Geometry: final body of the model. Coordinates: model frame, mm. Round coordinates to 2 decimals unless told otherwise and drop trailing zeros. Write each loop counter-clockwise with the first axis right and the second up, starting at its lowest first coordinate (ties: lowest second). Pieces come first, ordered by that corner, then holes. Notation, with made-up numbers: M 40.25,40.25 L 54.25,40.25 A29 ccw 54.25,70.25 Z; hole C 24.5,78.25 d9. An arc over 180 degrees is marked long. Use one line per item in the form item = value. Start each with the question number.
Item 1: Ray query, probe 1 along Y at (x, z) = (0, -18); probe 2 along Y at (x, z) = (0.25, 17); probe 3 along X at (y, z) = (0, -38.5). Return the intervals inside material, ascending.
Item 2: Section query A-A (z = 47). Return loops of the section in (x, y), and give its area (3 significant figures).
Item 3: Pin query (flat end, axial travel): pin 1 Ø4.5 at (x, y) = (0, 0) entering from -Z; pin 2 Ø1.6 at (x, y) = (-5.5, 4) entering from -Z (3 decimals); pin 3 Ø1.5 at (x, z) = (-3, 21.5) entering from -Y. Return the tip coordinate at first contact, or that it passes through.
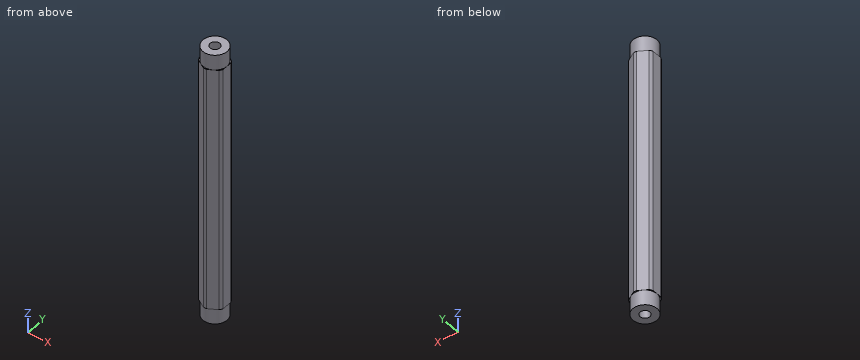
Autodesk Inventor part; units mm, degrees
ref_plane "YZ Plane" through (0, 0, 0) normal (1, 0, 0) x (0, 1, 0)
ref_plane "XZ Plane" through (0, 0, 0) normal (0, 1, 0) x (-1, 0, 0)
ref_plane "XY Plane" through (0, 0, 0) normal (0, 0, 1) x (1, 0, 0)
sketch "Sketch1" plane through (0, 0, 0) normal (0, 0, 1) x (1, 0, 0)
  line L0 (-6.35, -3.6662) -> (-6.35, 3.6662)
  line L1 (-6.35, 3.6662) -> (0, 7.3323)
  line L2 (0, 7.3323) -> (6.35, 3.6662)
  line L3 (6.35, 3.6662) -> (6.35, -3.6662)
  line L4 (6.35, -3.6662) -> (0, -7.3323)
  line L5 (0, -7.3323) -> (-6.35, -3.6662)
  point P0 (0, 0)
  point P1 (0, 0)
  dimension "Size" = 12.7
extrude "Extrusion1" add sketch "Sketch1" along normal mid plane 146.05
sketch "Sketch3" plane through (0, 0, 73.025) normal (0, 0, 1) x (1, 0, 0)
  line L0 (-6.35, 3.6662) -> (0, 7.3323) construction
  line L1 (0, 7.3323) -> (6.35, 3.6662) construction
  line L2 (6.35, 3.6662) -> (6.35, -3.6662) construction
  line L3 (6.35, -3.6662) -> (0, -7.3323) construction
  line L4 (0, -7.3323) -> (-6.35, -3.6662) construction
  line L5 (-6.35, -3.6662) -> (-6.35, 3.6662) construction
  point P0 (0, 0)
hole "Hole1" at (0, 0, 73.025) direction (0, 0, -1) diameter 5.1054 end through all
sketch "Sketch4" plane through (0, 0, 73.025) normal (0, 0, 1) x (1, 0, 0)
  circle A0 centre (0, 0) radius 2.5527 construction
  line L0 (-6.35, 3.6662) -> (0, 7.3323) construction
  line L1 (0, 7.3323) -> (6.35, 3.6662) construction
  line L2 (6.35, 3.6662) -> (6.35, -3.6662) construction
  line L3 (6.35, -3.6662) -> (0, -7.3323) construction
  line L4 (0, -7.3323) -> (-6.35, -3.6662) construction
  line L5 (-6.35, -3.6662) -> (-6.35, 3.6662) construction
  circle A1 centre (0, 0) radius 6.8771
  circle A2 centre (0, 0) radius 8.89
  dimension "thunder" = 13.7541
  dimension "d16" = 17.78
extrude "Extrusion3" cut sketch "Sketch4" against normal through all
sketch "Sketch5" plane through (0, 0, 73.025) normal (0, 0, 1) x (1, 0, 0)
  arc A0 (5.4616, -4.1791) -> (6.35, -2.6403) centre (0, 0) ccw
  line L0 (5.4616, -4.1791) -> (0.8884, -6.8194)
  arc A1 (-0.8884, -6.8194) -> (0.8884, -6.8194) centre (0, 0) ccw
  line L1 (-0.8884, -6.8194) -> (-5.4616, -4.1791)
  arc A2 (-6.35, -2.6403) -> (-5.4616, -4.1791) centre (0, 0) ccw
  line L2 (-6.35, -2.6403) -> (-6.35, 2.6403)
  arc A3 (-5.4616, 4.1791) -> (-6.35, 2.6403) centre (0, 0) ccw
  line L3 (-5.4616, 4.1791) -> (-0.8884, 6.8194)
  arc A4 (0.8884, 6.8194) -> (-0.8884, 6.8194) centre (0, 0) ccw
  line L4 (0.8884, 6.8194) -> (5.4616, 4.1791)
  arc A5 (6.35, 2.6403) -> (5.4616, 4.1791) centre (0, 0) ccw
  line L5 (6.35, 2.6403) -> (6.35, -2.6403)
  circle A6 centre (0, 0) radius 2.5527
  circle A7 centre (0, 0) radius 6.35
  point P0 (-3.175, 5.4993)
  point P1 (3.175, 5.4993)
  point P2 (6.35, 0)
  point P3 (-6.35, 0)
  point P4 (-3.175, -5.4993)
  point P5 (3.175, -5.4993)
  dimension "d19" = 12.7
extrude "Extrusion4" cut sketch "Sketch5" against normal blind 8.001 contours L0 A7 L5 A0 | L0 A1 L1 A7 | A7 L4 A5 L5 | L1 A2 L2 A7 | A7 L3 A4 L4 | L2 A3 L3 A7
mirror "Mirror2" about plane through (0, 0, 0) normal (0, 0, 1) of "Extrusion4"
equation "\"bearing\" = 25.4"
properties part number "CL4-019" material "Aluminum 6061"
Working result:
q1.probe_1 = -6.88 to -2.55, 2.55 to 6.88
q1.probe_2 = -6.87 to -2.54, 2.54 to 6.87
q1.probe_3 = -6.35 to -2.55, 2.55 to 6.35
q2.outline = M -6.35,-2.64 A6.88 ccw -5.46,-4.18 L -0.89,-6.82 A6.88 ccw 0.89,-6.82 L 5.46,-4.18 A6.88 ccw 6.35,-2.64 L 6.35,2.64 A6.88 ccw 5.46,4.18 L 0.89,6.82 A6.88 ccw -0.89,6.82 L -5.46,4.18 A6.88 ccw -6.35,2.64 Z; hole C 0,0 d5.11
q2.area = 117 mm²
q3.pin_1 = through
q3.pin_2 = -73.025
q3.pin_3 = -6.03
